Part model, mm, in its own coordinate system. A direction names the side the tool comes from. Give positions to 0.01 mm unless a question says otherwise; leave off trailing zeros. Write each loop counter-clockwise with the first axis right and the second up, starting at its lowest first coordinate (ties: lowest second). Pieces come first, ordered by that corner, then holes. Notation, with made-up numbers: M 54.5,48 L 106.5,48 A24 cw 106.5,80 Z; hole C 32.5,82.5 d2. An arc over 180 degrees is marked long. Use a Markdown table: item, result.
```python
from build123d import *

# Parameters (mm, degrees)
F0_W     = 444.5
F0_H     = 406.4
F0_W_2   = 419.1
F0_H_2   = 381
F1_DEPTH = 63.5
F2_W     = 419.1
F2_H     = 381
F3_DEPTH = 12.7
F4_W     = 419.1
F4_H     = 381
F5_DEPTH = 6.35
F6_W     = 50.8
F6_H     = 19.05
F7_DEPTH = 25.4


with BuildPart() as f1:
    # F0 (on Top) → F1 (new body)
    with BuildSketch(Plane.XY):
        Rectangle(F0_W, F0_H)
        Rectangle(F0_W_2, F0_H_2, mode=Mode.SUBTRACT)
    extrude(amount=F1_DEPTH)

    # F2 (on face) → F3 (join)
    with BuildSketch(Plane(origin=(0, 0, 0), x_dir=(1, 0, 0), z_dir=(0, 0, -1))):
        Rectangle(F2_W, F2_H)
    extrude(amount=-F3_DEPTH)

    # F4 (on face) → F5 (cut)
    with BuildSketch(Plane(origin=(0, 0, 0), x_dir=(1, 0, 0), z_dir=(0, 0, -1))):
        Rectangle(F4_W, F4_H)
    extrude(amount=-F5_DEPTH, mode=Mode.SUBTRACT)

    # F6 (on face) → F7 (cut)
    with BuildSketch(Plane.XZ.offset(203.2)):
        with Locations((171.45, 53.975)):
            Rectangle(F6_W, F6_H)
    extrude(amount=-F7_DEPTH, mode=Mode.SUBTRACT)


solid = f1.part
```
1. Drop flat-ended pins along their axis: P1, Ø10, axis at x = 122, y = -140.5, coming from the +Z side; P2, Ø10, axis at x = 169, y = -197, coming from the +Z side; P3, Ø1, axis at x = 55, y = -76, coming from the -Z side. Give the stop position or say it passes through.
Findings below:
| item | result |
|---|---|
| P1 | z = 12.7 |
| P2 | z = 44.45 |
| P3 | z = 6.35 |
2. Cut at C-C, the plane z = 31.5. Give the cut face in (x, y).
Findings below:
| item | result |
|---|---|
| outline | M -222.25,-203.2 L 222.25,-203.2 L 222.25,203.2 L -222.25,203.2 Z; hole M -209.55,-190.5 L 209.55,-190.5 L 209.55,190.5 L -209.55,190.5 Z |
3. Drill centre lines: L1, parallel to X at y = -173.5, z = 24.5; L2, parallel to Y at x = -12, z = 32.5; L3, parallel to Z at x = 194, y = 146. Where is each one in solid material? Low to high.
Findings below:
| item | result |
|---|---|
| L1 | -222.25 to -209.55, 209.55 to 222.25 |
| L2 | -203.2 to -190.5, 190.5 to 203.2 |
| L3 | 6.35 to 12.7 |
4. Two-plate mould, pull along Y, no slides. Class faces 1 (the flat face through (-3, 203.2, 31)), 2 (the flat face through (171, -197, 44.45)), 3 (the flat face through (-3, 190.5, 38)), 4 (the flat face through (-3, -3, 12.7)): released by +Y, released by -Y, zero draft, split by the parting line, or undercut.
Findings below:
| item | result |
|---|---|
| face 1 | released by +Y |
| face 2 | zero draft |
| face 3 | undercut |
| face 4 | undercut |
5. Tool access for faces 5 (the flat face through (-3, -203.2, 31)), 6 (the flat face through (-3, -3, 6.35)), 7 (the flat face through (-209.55, -3, 38)), 8 (the flat face through (-18, 195, 0)), 9 (the flat face through (196.85, -197, 54)): list every direction of +Z, -Z, +X, -X, +Y, -Y with a clear straight run to the whole face (end or side of a thin tool).
Findings below:
| item | result |
|---|---|
| face 5 | +Z, -Z, +X, -X, -Y |
| face 6 | -Z |
| face 7 | +Z |
| face 8 | -Z, +X, -X, +Y, -Y |
| face 9 | +Z, -Y |
6. Cut at A-A, the plane y = 90.5. Give the cut face in (x, z).
Findings below:
| item | result |
|---|---|
| outline | M -222.25,0 L -209.55,0 L -209.55,6.35 L 209.55,6.35 L 209.55,0 L 222.25,0 L 222.25,63.5 L 209.55,63.5 L 209.55,12.7 L -209.55,12.7 L -209.55,63.5 L -222.25,63.5 Z |
7. Cut at B-B, the plane x = 189. Give the cut face in (y, z), then the cut area to 3 significant figures.
Findings below:
| item | result |
|---|---|
| outline | M -203.2,0 L -190.5,0 L -190.5,6.35 L 190.5,6.35 L 190.5,0 L 203.2,0 L 203.2,63.5 L 190.5,63.5 L 190.5,12.7 L -190.5,12.7 L -190.5,44.45 L -203.2,44.45 Z |
| area | 3,790 mm2 |
